Geometry check sheet. Reference: drawing and pictorial views, mm from the part's lowest x, y, z. A direction names the side the tool comes from. Round coordinates to 2 decimals unless told otherwise and drop trailing zeros. Order: outer loops, then holes, each group sorted by start corner. A loop starts at its lowest first (then second) coordinate and runs counter-clockwise, first axis right, second up.
Q1. Cross-section at C-C on z = 35. Record the cut outline in (x, y), then the cut area to 3 significant figures.
Q2. Scan lines: probe 1 along Y at (x, z) = (24.5, 40); probe 2 along Z at (x, y) = (21, 40). Record each from-to range of solid material in increasing order.
Q3. Cross-section at B-B on x = 78. Record the cut outline in (y, z).
Q4. Cross-section at D-D on x = 45. Record the cut outline in (y, z), then the cut area to 3 significant figures.
Q5. Set-up check for the marked faces 1, 2 and 3: record each of +Z, -Z, +X, -X, +Y, -Y from which the full face is reachable in a straight line by a thin tool's end or side.
Q6. Mould release check, pull along Y, two halves, no side actions. Record for the marked faces 4, 5 and 6: +Y half, -Y half, draft (parallel to the pull), parting line (faces both ways), or undercut.
Q7. Depth check by flat-ended pin: P1, Ø4.5, axis at y = 70, z = 41.5, coming from the -X side; P2, Ø24, axis at x = 82, y = 61, coming from the +Z side; P3, Ø8, axis at x = 43.5, y = 12.5, coming from the -Z side; P4, Ø12, axis at x = 37.5, z = 46.5, coming from the +Y side. Enter the tip coordinate at first touch or a pass-through.
Q8. Cross-section at A-A on y = 32. Record the cut outline in (x, z), then the cut area to 3 significant figures.
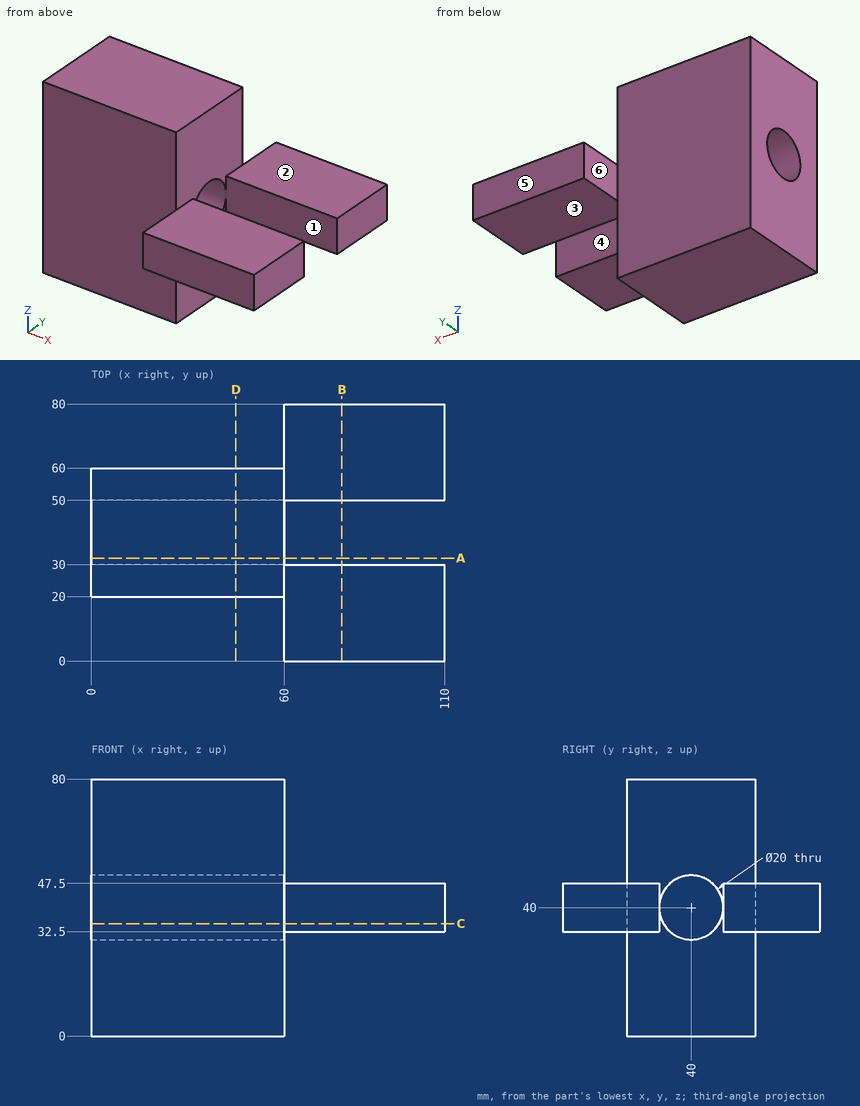
Results found:
1. outline: (0, 20) - (60, 20) - (60, 0) - (110, 0) - (110, 30) - (60, 30) - (60, 31.34) - (0, 31.34) - close; (0, 48.66) - (60, 48.66) - (60, 50) - (110, 50) - (110, 80) - (60, 80) - (60, 60) - (0, 60) - close
1. area: 4,360 mm2
2. probe 1: y = 20 to 30, 50 to 60
2. probe 2: z = 0 to 30, 50 to 80
3. outline: (0, 32.5) - (30, 32.5) - (30, 47.5) - (0, 47.5) - close; (50, 32.5) - (80, 32.5) - (80, 47.5) - (50, 47.5) - close
4. outline: (20, 0) - (60, 0) - (60, 80) - (20, 80) - close; hole circle Ø20 at (40, 40)
4. area: 2,890 mm2
5. face 1: +Z, -Z, +X
5. face 2: +Z, +X, +Y, -Y
5. face 3: -Z, +X, +Y, -Y
6. face 4: undercut
6. face 5: +Y half
6. face 6: draft
7. P1: stops at x = 60
7. P2: stops at z = 47.5
7. P3: passes through
7. P4: stops at y = 60
8. outline: (0, 0) - (60, 0) - (60, 34) - (0, 34) - close; (0, 46) - (60, 46) - (60, 80) - (0, 80) - close
8. area: 4,080 mm2
